Design review of the part built by this model. Coordinates are the model's own, in mm. A direction names the side the tool comes from. Coordinates: 2 decimals unless noted, no trailing zeros. Write item = value, one per line. Start each with the question number.
```python
from build123d import *

# Parameters (mm, degrees)
BOSS_EXTRUDE1_DEPTH     = 70
CUT_EXTRUDE1_DEPTH      = 72.414284285
CUT_EXTRUDE1_DEPTH_BACK = 72.414284285
SKETCH3_R               = 2


# Read off the part's stored shape, not the designer's step: Imported1
with BuildPart() as part:
    # Sketch1 → Boss-Extrude1 (new body)
    with BuildSketch(Plane(origin=(0, 0, 0), x_dir=(1, 0, 0), z_dir=(0, 1, 0))):
        with BuildLine():
            Line((4.5, -0.866025), (4, 0))
            Line((4, 0), (4.5, 0.866025))
            Line((4.5, 0.866025), (4.5, 3.43934))
            Line((4.5, 3.43934), (7.06066, 6))
            Line((7.06066, 6), (8.5, 6))
            Line((8.5, 6), (8.5, 3))
            Line((8.5, 3), (9.5, 3))
            Line((9.5, 3), (9.5, 3.5))
            Line((9.5, 3.5), (10, 3.5))
            Line((10, 3.5), (10, 8.5))
            ThreePointArc((10, 8.5), (9.560660172, 9.560660172), (8.5, 10))
            Line((8.5, 10), (3.5, 10))
            Line((3.5, 10), (3.5, 9.5))
            Line((3.5, 9.5), (3, 9.5))
            Line((3, 9.5), (3, 8.5))
            Line((3, 8.5), (6, 8.5))
            Line((6, 8.5), (6, 7.06066))
            Line((6, 7.06066), (3.43934, 4.5))
            Line((3.43934, 4.5), (0.866025, 4.5))
            Line((0.866025, 4.5), (0, 4))
            Line((0, 4), (-0.866025, 4.5))
            Line((-0.866025, 4.5), (-3.43934, 4.5))
            Line((-3.43934, 4.5), (-6, 7.06066))
            Line((-6, 7.06066), (-6, 8.5))
            Line((-6, 8.5), (-3, 8.5))
            Line((-3, 8.5), (-3, 9.5))
            Line((-3, 9.5), (-3.5, 9.5))
            Line((-3.5, 9.5), (-3.5, 10))
            Line((-3.5, 10), (-8.5, 10))
            ThreePointArc((-8.5, 10), (-9.560660172, 9.560660172), (-10, 8.5))
            Line((-10, 8.5), (-10, 3.5))
            Line((-10, 3.5), (-9.5, 3.5))
            Line((-9.5, 3.5), (-9.5, 3))
            Line((-9.5, 3), (-8.5, 3))
            Line((-8.5, 3), (-8.5, 6))
            Line((-8.5, 6), (-7.06066, 6))
            Line((-7.06066, 6), (-4.5, 3.43934))
            Line((-4.5, 3.43934), (-4.5, 0.866025))
            Line((-4.5, 0.866025), (-4, 0))
            Line((-4, 0), (-4.5, -0.866025))
            Line((-4.5, -0.866025), (-4.5, -3.43934))
            Line((-4.5, -3.43934), (-7.06066, -6))
            Line((-7.06066, -6), (-8.5, -6))
            Line((-8.5, -6), (-8.5, -3))
            Line((-8.5, -3), (-9.5, -3))
            Line((-9.5, -3), (-9.5, -3.5))
            Line((-9.5, -3.5), (-10, -3.5))
            Line((-10, -3.5), (-10, -8.5))
            ThreePointArc((-10, -8.5), (-9.560660172, -9.560660172), (-8.5, -10))
            Line((-8.5, -10), (-3.5, -10))
            Line((-3.5, -10), (-3.5, -9.5))
            Line((-3.5, -9.5), (-3, -9.5))
            Line((-3, -9.5), (-3, -8.5))
            Line((-3, -8.5), (-6, -8.5))
            Line((-6, -8.5), (-6, -7.06066))
            Line((-6, -7.06066), (-3.43934, -4.5))
            Line((-3.43934, -4.5), (-0.866025, -4.5))
            Line((-0.866025, -4.5), (0, -4))
            Line((0, -4), (0.866025, -4.5))
            Line((0.866025, -4.5), (3.43934, -4.5))
            Line((3.43934, -4.5), (6, -7.06066))
            Line((6, -7.06066), (6, -8.5))
            Line((6, -8.5), (3, -8.5))
            Line((3, -8.5), (3, -9.5))
            Line((3, -9.5), (3.5, -9.5))
            Line((3.5, -9.5), (3.5, -10))
            Line((3.5, -10), (8.5, -10))
            ThreePointArc((8.5, -10), (9.560660172, -9.560660172), (10, -8.5))
            Line((10, -8.5), (10, -3.5))
            Line((10, -3.5), (9.5, -3.5))
            Line((9.5, -3.5), (9.5, -3))
            Line((9.5, -3), (8.5, -3))
            Line((8.5, -3), (8.5, -6))
            Line((8.5, -6), (7.06066, -6))
            Line((7.06066, -6), (4.5, -3.43934))
            Line((4.5, -3.43934), (4.5, -0.866025))
        make_face()
        with BuildLine():
            Line((2.947757456, -1.8869899), (2.435674593, -1.276711693))
            ThreePointArc((2.435674593, -1.276711693), (2.750000433, -2.31e-07), (2.435674303, 1.276711159))
            Line((2.435674303, 1.276711159), (2.947757255, 1.886989128))
            ThreePointArc((2.947757255, 1.886989128), (2.474929059, 2.474818349), (1.887120795, 2.947672597))
            Line((1.887120795, 2.947672597), (1.276854759, 2.435598541))
            ThreePointArc((1.276854759, 2.435598541), (-1.33e-07, 2.749999412), (-1.276854885, 2.435597973))
            Line((-1.276854885, 2.435597973), (-1.887121068, 2.94767181))
            ThreePointArc((-1.887121068, 2.94767181), (-2.47492916, 2.474817292), (-2.947757123, 1.886987839))
            Line((-2.947757123, 1.886987839), (-2.43567406, 1.276709798))
            ThreePointArc((-2.43567406, 1.276709798), (-2.749999477, -6.08e-07), (-2.435674, -1.276711))
            Line((-2.435674, -1.276711), (-2.947757054, -1.886989034))
            ThreePointArc((-2.947757054, -1.886989034), (-2.474929075, -2.474818464), (-1.887120973, -2.947672958))
            Line((-1.887120973, -2.947672958), (-1.276855, -2.435599))
            ThreePointArc((-1.276855, -2.435599), (-1.15e-07, -2.750000499), (1.276854906, -2.43559955))
            Line((1.276854906, -2.43559955), (1.887120935, -2.947673594))
            ThreePointArc((1.887120935, -2.947673594), (2.47492925, -2.474819245), (2.947757456, -1.8869899))
        make_face(mode=Mode.SUBTRACT)
    extrude(amount=BOSS_EXTRUDE1_DEPTH)

    # Sketch3 → Cut-Extrude1 (cut, two sides: drawn at the far end of the back side and taken through both)
    with BuildSketch(Plane.XY.offset(-CUT_EXTRUDE1_DEPTH_BACK)):
        with Locations(Location((0, 8, 0), (0, 0, 340.658342389))):
            Circle(SKETCH3_R)
        Polygon((-10, 6), (-4, 0), (-10, 0), align=None)
        Polygon((10, 0), (10, 6), (4, 0), align=None)
    extrude(amount=CUT_EXTRUDE1_DEPTH + CUT_EXTRUDE1_DEPTH_BACK, mode=Mode.SUBTRACT)


solid = part.part
```
(1) Mouldability with a two-part tool opening along X and no side actions: class faces 1 (the flat face through (-6, 36, -8)), 2 (the flat face through (-7, 3, 7)), 3 (the flat face through (-6, 36, 8)), 4 (the flat face through (6, 35, -10)) as +X half, -X half, draft (parallel to the pull), parting line (faces both ways), or undercut.
(2) Insertion check: pin 1 (0.8 mm diameter, centred on y = 39, z = 9, fed in from +X); pin 2 (4.5 mm diameter, centred on x = 0, y = 8, fed in from -Z). Each pin has a flat end and moves straight along its axis. Give the tip position at first contact, or say it passes through.
(3) Tool access review of faces 5 (the flat face through (4.74, 34.51, -5.8)), 6 (the flat face through (2, 70, 4)): name each direction out of +Z, -Z, +X, -X, +Y, -Y from which nothing blocks a thin tool from reaching the whole face with its end or side.
(4) To check wall thickness, follow L1, parallel to X at y = 8, z = -3.4; L2, parallel to Y at x = 0, z = 3.65; L3, parallel to X at y = 8, z = 4. State the ranges of each line that lie inside material, in increasing order.
Results list:
q1.face_1 = undercut
q1.face_2 = -X half
q1.face_3 = undercut
q1.face_4 = draft
q2.pin_1 = 10
q2.pin_2 = -4.5
q3.face_5 = +Y, -Y
q3.face_6 = +Z, -Z, +X, -X, +Y
q4.L1 = -9.5 to -8.5, -4.5 to -2, 2 to 4.5, 8.5 to 9.5
q4.L2 = 0 to 6, 10 to 70
q4.L3 = -10 to -8.5, -5.06 to -2, 2 to 5.06, 8.5 to 10
